Verification items for the finished model (mm, model axes). Face numbers are marked on the shaded views. A direction names the side the tool comes from. Round coordinates to 2 decimals unless told otherwise and drop trailing zeros. Write each loop counter-clockwise with the first axis right and the second up, starting at its lowest first coordinate (ties: lowest second). Pieces come first, ordered by that corner, then holes. Notation, with made-up numbers: (44, -5) - (97, -5) arc R29 cw to (97, 21) - close; hole circle Ø6 at (-24.75, -40). An arc over 180 degrees is marked (long way). Answer as a JSON object with one key per item and string values.
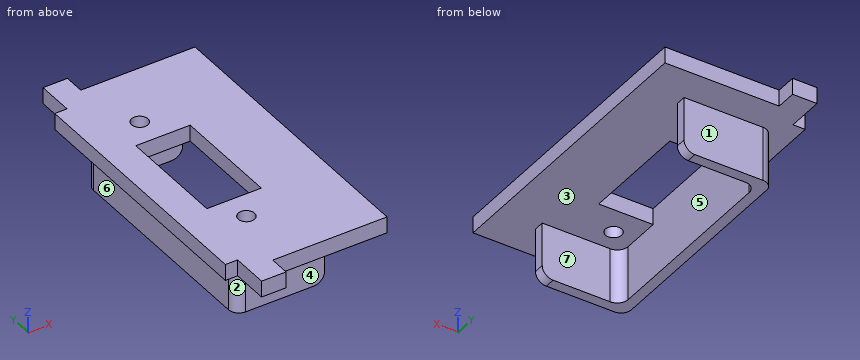
Autodesk Inventor part; units mm, degrees
ref_plane "YZ Plane" through (0, 0, 0) normal (1, 0, 0) x (0, 1, 0)
ref_plane "XZ Plane" through (0, 0, 0) normal (0, 1, 0) x (-1, 0, 0)
ref_plane "XY Plane" through (0, 0, 0) normal (0, 0, 1) x (1, 0, 0)
ref_plane "Work Plane1" through (0, 0, 0) normal (0, 0, 1) x (1, 0, 0)
sketch "Sketch1" plane through (0, 0, 0) normal (0, 0, 1) x (1, 0, 0)
  line L0 (0, 0) -> (23.25, 0)
  line L1 (0, -48) -> (0, 0)
  line L2 (23.25, -48) -> (0, -48)
  line L3 (23.25, -48) -> (23.25, -31.5)
  line L4 (23.25, -31.5) -> (26.25, -31.5)
  line L5 (27.75, -30) -> (26.25, -31.5)
  line L6 (27.75, -30) -> (27.75, -18)
  line L7 (27.75, -18) -> (26.25, -16.5)
  line L8 (23.25, -16.5) -> (26.25, -16.5)
  line L9 (23.25, 0) -> (23.25, -16.5)
  line L10 (20.25, -16.5) -> (20.25, -3)
  line L11 (17.25, -16.5) -> (20.25, -16.5)
  line L12 (17.25, -16.5) -> (17.25, -19.5)
  line L13 (26.25, -19.5) -> (26.25, -28.5)
  line L14 (17.25, -28.5) -> (17.25, -31.5)
  line L15 (17.25, -31.5) -> (20.25, -31.5)
  line L16 (20.25, -31.5) -> (20.25, -45)
  line L17 (3.75, -45) -> (20.25, -45)
  line L18 (3.75, -3) -> (3.75, -45)
  line L19 (20.25, -3) -> (3.75, -3)
  line L20 (17.25, -19.5) -> (17.25, -28.5)
  line L21 (18.25, -33.5) -> (15.25, -33.5)
  line L22 (15.25, -33.5) -> (15.25, -28.5)
  line L23 (15.25, -28.5) -> (15.25, -19.5)
  line L24 (15.25, -19.5) -> (15.25, -14.5)
  line L25 (15.25, -14.5) -> (18.25, -14.5)
  line L26 (20.25, -5) -> (5.75, -5)
  line L27 (5.75, -5) -> (5.75, -43)
  line L28 (5.75, -43) -> (20.25, -43)
extrude "Extrusion1" add sketch "Sketch1" against normal blind 10 contours L26 L27 L28 L16 L17 L18 L19 L10
sketch "Sketch2" plane through (0, 0, 0) normal (0, 0, 1) x (1, 0, 0)
  line L0 (2.25, 0) -> (2.25, 6.75)
  line L1 (2.25, 0) -> (3.3, 0)
  line L2 (3.3, 0) -> (3.3, 5.7)
  line L3 (5.7, 5.7) -> (3.3, 5.7)
  line L4 (5.7, 1.95) -> (5.7, 5.7)
  line L5 (26.7, 1.95) -> (5.7, 1.95)
  line L6 (26.7, 1.95) -> (26.7, -16.95)
  line L7 (26.7, -16.95) -> (27.75, -18)
  line L8 (27.75, -18) -> (27.75, 3)
  line L9 (6.75, 3) -> (27.75, 3)
  line L10 (6.75, 3) -> (6.75, 6.75)
  line L11 (2.25, 6.75) -> (6.75, 6.75)
  line L12 (2.25, -54.75) -> (2.25, -48)
  line L13 (2.25, -54.75) -> (6.75, -54.75)
  line L14 (6.75, -54.75) -> (6.75, -51)
  line L15 (6.75, -51) -> (27.75, -51)
  line L16 (27.75, -51) -> (27.75, -30)
  line L17 (26.7, -31.05) -> (27.75, -30)
  line L18 (26.7, -31.05) -> (26.7, -49.95)
  line L19 (26.7, -49.95) -> (5.7, -49.95)
  line L20 (5.7, -49.95) -> (5.7, -53.7)
  line L21 (3.3, -53.7) -> (5.7, -53.7)
  line L22 (3.3, -53.7) -> (3.3, -48)
  line L23 (2.25, -48) -> (3.3, -48)
  line L24 (0, 0) -> (23.25, 0)
  line L25 (0, -48) -> (0, 0)
  line L26 (23.25, -48) -> (0, -48)
  line L27 (23.25, -48) -> (23.25, -31.5)
  line L28 (23.25, -31.5) -> (26.25, -31.5)
  line L29 (27.75, -30) -> (26.25, -31.5)
  line L30 (27.75, -30) -> (27.75, -18)
  line L31 (27.75, -18) -> (26.25, -16.5)
  line L32 (23.25, -16.5) -> (26.25, -16.5)
  line L33 (23.25, 0) -> (23.25, -16.5)
  line L34 (20.25, -16.5) -> (20.25, -3)
  line L35 (17.25, -16.5) -> (20.25, -16.5)
  line L36 (17.25, -16.5) -> (17.25, -19.5)
  line L37 (17.25, -19.5) -> (26.25, -19.5)
  line L38 (26.25, -19.5) -> (26.25, -28.5)
  line L39 (17.25, -28.5) -> (26.25, -28.5)
  line L40 (17.25, -28.5) -> (17.25, -31.5)
  line L41 (17.25, -31.5) -> (20.25, -31.5)
  line L42 (20.25, -31.5) -> (20.25, -45)
  line L43 (3.75, -45) -> (20.25, -45)
  line L44 (3.75, -3) -> (3.75, -45)
  line L45 (20.25, -3) -> (3.75, -3)
extrude "Extrusion2" add sketch "Sketch2" along normal blind 3 contours L0 L11 L10 L9 L8 L7 L6 L5 L4 L3 L2 L1 | L1 L24 L33 L32 L31 L7 L30 L17 L29 L28 L27 L26 L23 L25 | L2 L3 L4 L5 L6 L31 L32 L33 L24 | L23 L22 L21 L20 L19 L18 L17 L16 L15 L14 L13 L12 | L26 L27 L28 L29 L18 L19 L20 L21 L22 | L35 L36 L37 L38 L39 L40 L41 L42 L43 L44 L45 L34
sketch "Sketch3" plane through (0, 0, 0) normal (0, 0, -1) x (-1, 0, 0)
  line L0 (-5.75, -34) -> (-15.75, -34)
  line L1 (-15.75, -34) -> (-15.75, -14)
  line L2 (-15.75, -14) -> (-5.75, -14)
  line L3 (-5.75, -14) -> (-5.75, -34)
  line L4 (-3.75, -45) -> (-3.75, -3) construction
  line L5 (-3.75, -24) -> (-33.6662, -24) construction
  line L6 (-5.75, -5) -> (-5.75, -43) construction
  point P0 (0, 0)
  dimension "d5" = 10
  dimension "d6" = 20
extrude "Extrusion3" cut sketch "Sketch3" against normal through all
sketch "Sketch4" plane through (0, 0, 0) normal (0, 0, -1) x (-1, 0, 0)
  line L0 (-20.25, -5) -> (-5.75, -5)
  line L1 (-5.75, -43) -> (-20.25, -43)
  line L2 (-5.75, -5) -> (-5.75, -43)
  point P0 (0, 0)
  point P1 (-9.75, -9)
  point P2 (-9.75, -39)
  dimension "d9" = 4
  dimension "d10" = 4
  dimension "d11" = 4
  dimension "d12" = 4
hole "Hole1" at (9.75, -9, 0) at (9.75, -39, 0) direction (0, 0, 1) diameter 3 end through all
fillet "Fillet1" radius 2 6 edges at (20.25, -4, -10) (20.25, -44, -10) (3.75, -3, -5) (3.75, -45, -5) (5.75, -43, -5) (5.75, -5, -5)
thicken "Thicken1" operation add thickness 0.1 both sides no extend neighbours yes toward (0, 1, 0) faces at (14.75, -45, -3.3333) (4.75, -44.732, -3.3333) (3.75, -17.6667, -3.3333) (4.2839, -3.6397, -3.3333) (14.75, -3, -3.3333)
properties part number "camera_holder"
1. Go/stop test with flat-tipped pins: pin 1 (2 mm diameter, centred on y = -8.5, z = -1.5, fed in from -X); pin 2 (0.9 mm diameter, centred on y = -52.5, z = 2, fed in from -X); pin 3 (1.5 mm diameter, centred on y = -38, z = -3, fed in from +X). Record where each tip stops, or that it passes through.
Completed:
{"pin 1": "stops at x = 3.85", "pin 2": "stops at x = 2.25", "pin 3": "stops at x = 5.75"}
2. Cross-section at C-C (z = 1.75). Record the boundary of the cut face in (x, y), plus the area to 3 significant figures.
Completed:
{"outline": "(0, -48) - (2.25, -48) - (2.25, -54.75) - (6.75, -54.75) - (6.75, -51) - (27.75, -51) - (27.75, 3) - (6.75, 3) - (6.75, 6.75) - (2.25, 6.75) - (2.25, 0) - (0, 0) - close; hole (5.75, -34) - (15.75, -34) - (15.75, -14) - (5.75, -14) - close; hole circle Ø3 at (9.75, -39); hole circle Ø3 at (9.75, -9)", "area": "1,300 mm^2"}
3. Material ranges on probe 1 along Y at (x, z) = (9.75, 2.25); probe 2 along Y at (x, z) = (15.5, 2.75); probe 3 along Y at (x, z) = (9.25, -1), recorded low to high. Write a range as from..to.
Completed:
{"probe 1": "y = -51..-40.5, -37.5..-34, -14..-10.5, -7.5..3", "probe 2": "y = -51..-34, -14..3", "probe 3": "y = -44.9..-43, -5..-3.1"}
4. Access from +Z, -Z, +X, -X, +Y, -Y to the whole of each face (thin tool, end or side, straight path). Record for the marked faces 4, 5, 6 and 7.
Completed:
{"face 4": "-Z, +X, -X, -Y", "face 5": "-Z", "face 6": "-Z, -X, +Y, -Y", "face 7": "-Z, +X"}
5. Mould release check, pull along Y, two halves, no side actions. Record for the marked faces 1, 2 and 3: released by +Y, released by -Y, zero draft, split by the parting line, or undercut.
Completed:
{"face 1": "released by +Y", "face 2": "released by -Y", "face 3": "undercut"}
6. Cross-section at B-B (y = -9). Record the boundary of the cut face in (x, z), plus the area to 4 significant figures.
Completed:
{"outline": "(0, 0) - (3.85, 0) - (3.85, -10) - (5.75, -10) - (5.75, 0) - (8.25, 0) - (8.25, 3) - (0, 3) - close; (11.25, 0) - (27.75, 0) - (27.75, 3) - (11.25, 3) - close", "area": "93.25 mm^2"}
7. Cross-section at D-D (x = 12.75). Record the boundary of the cut face in (y, z).
Completed:
{"outline": "(-51, 0) - (-44.9, 0) - (-44.9, -10) - (-43, -10) - (-43, 0) - (-34, 0) - (-34, 3) - (-51, 3) - close; (-14, 0) - (-5, 0) - (-5, -10) - (-3.1, -10) - (-3.1, 0) - (3, 0) - (3, 3) - (-14, 3) - close"}
8. Cross-section at A-A (x = 9.75). Record the boundary of the cut face in (y, z).
Completed:
{"outline": "(-51, 0) - (-44.9, 0) - (-44.9, -10) - (-43, -10) - (-43, 0) - (-40.5, 0) - (-40.5, 3) - (-51, 3) - close; (-37.5, 0) - (-34, 0) - (-34, 3) - (-37.5, 3) - close; (-14, 0) - (-10.5, 0) - (-10.5, 3) - (-14, 3) - close; (-7.5, 0) - (-5, 0) - (-5, -10) - (-3.1, -10) - (-3.1, 0) - (3, 0) - (3, 3) - (-7.5, 3) - close"}
